```python
from build123d import *

# Parameters (mm, degrees)
F0_R     = 1.05
F1_DEPTH = 3


with BuildPart() as f1:
    # F0 (on Top) → F1 (new body)
    with BuildSketch(Plane.XY):
        with BuildLine():
            Line((-31, -43.5), (-33.75, -43.5))
            ThreePointArc((-33.75, -43.5), (-36.5, -46.25), (-33.75, -49))
            Line((-33.75, -49), (33.75, -49))
            ThreePointArc((33.75, -49), (36.5, -46.25), (33.75, -43.5))
            Line((33.75, -43.5), (31, -43.5))
            Line((31, -43.5), (31, 43.5))
            Line((31, 43.5), (32.5, 43.5))
            ThreePointArc((32.5, 43.5), (35.25, 46.25), (32.5, 49))
            Line((32.5, 49), (-32.5, 49))
            ThreePointArc((-32.5, 49), (-35.25, 46.25), (-32.5, 43.5))
            Line((-32.5, 43.5), (-31, 43.5))
            Line((-31, 43.5), (-31, -43.5))
        make_face()
        with Locations((-33.75, -46.25)):
            Circle(F0_R, mode=Mode.SUBTRACT)
        with Locations((33.75, -46.25)):
            Circle(F0_R, mode=Mode.SUBTRACT)
        with Locations((-32.5, 46.25)):
            Circle(F0_R, mode=Mode.SUBTRACT)
        with Locations((32.5, 46.25)):
            Circle(F0_R, mode=Mode.SUBTRACT)
    extrude(amount=F1_DEPTH)


solid = f1.part
```
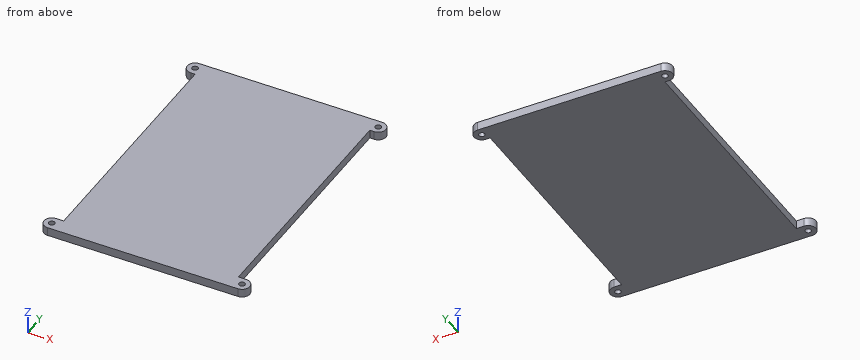
Input: part model. Units: mm. Frame: model coordinates. Give positions to 0.01 mm unless a question says otherwise; leave off trailing zeros. Order: outer loops, then holes, each group sorted by start corner. A loop starts at its lowest first (then second) coordinate and runs counter-clockwise, first axis right, second up.
1. Cut plane A-A (y = -46.25). Return loops of the section in (x, z), and give its area (3 significant figures).
Computed:
outline: (-36.5, 0) - (-34.8, 0) - (-34.8, 3) - (-36.5, 3) - close; (-32.7, 0) - (32.7, 0) - (32.7, 3) - (-32.7, 3) - close; (34.8, 0) - (36.5, 0) - (36.5, 3) - (34.8, 3) - close
area: 206 mm2
2. Pin query (flat end, axial travel): pin 1 Ø1.5 at (y, z) = (-17.5, 2) entering from -X. Return the tip coordinate at first contact, or that it passes through.
Computed:
pin 1: stops at x = -31
3. Cut plane D-D (y = -19). Return loops of the section in (x, z).
Computed:
outline: (-31, 0) - (31, 0) - (31, 3) - (-31, 3) - close
4. Line query: probe 1 along Y at (x, z) = (32.5, 2.15); probe 2 along Y at (x, z) = (-33, 2.55); probe 3 along Y at (x, z) = (-33.75, 0.7). Output: solid intervals per line, ascending.
Computed:
probe 1: y = -49 to -43.5, 43.5 to 45.2, 47.3 to 49
probe 2: y = -49 to -46.98, -45.52 to -43.5, 43.55 to 45.33, 47.17 to 48.95
probe 3: y = -49 to -47.3, -45.2 to -43.5, 43.8 to 48.7
5. Cut plane B-B (z = 1.45). Return loops of the section in (x, y).
Computed:
outline: (-33.75, -49) - (33.75, -49) arc R2.75 ccw to (33.75, -43.5) - (31, -43.5) - (31, 43.5) - (32.5, 43.5) arc R2.75 ccw to (32.5, 49) - (-32.5, 49) arc R2.75 ccw to (-32.5, 43.5) - (-31, 43.5) - (-31, -43.5) - (-33.75, -43.5) arc R2.75 ccw to start; hole circle Ø2.1 at (-33.75, -46.25); hole circle Ø2.1 at (-32.5, 46.25); hole circle Ø2.1 at (32.5, 46.25); hole circle Ø2.1 at (33.75, -46.25)
6. Cut plane C-C (y = 46.25). Return loops of the section in (x, z).
Computed:
outline: (-35.25, 0) - (-33.55, 0) - (-33.55, 3) - (-35.25, 3) - close; (-31.45, 0) - (31.45, 0) - (31.45, 3) - (-31.45, 3) - close; (33.55, 0) - (35.25, 0) - (35.25, 3) - (33.55, 3) - close
